```python
from build123d import *

# Parameters (mm, degrees)
SKETCH1_W           = 50.8
SKETCH1_H           = 39.878
BOSS_EXTRUDE1_DEPTH = 53.499926347
SKETCH3_W           = 43.18
SKETCH3_H           = 50.8
CUT_EXTRUDE1_DEPTH  = 30.353
CUT_EXTRUDE2_DEPTH  = 51.8
FILLET3_R           = 2.54
FILLET4_R           = 2.54
FILLET5_R           = 2.54
SKETCH5_R           = 3.175
CUT_EXTRUDE3_DEPTH  = 6.08
CUT_EXTRUDE4_DEPTH  = 25.4


with BuildPart() as part:
    # Sketch1 → Boss-Extrude1 (new body)
    with BuildSketch(Plane(origin=(0, 0, 0), x_dir=(1, 0, 0), z_dir=(0, 1, 0))):
        with Locations((25.4, 19.939)):
            Rectangle(SKETCH1_W, SKETCH1_H)
    extrude(amount=BOSS_EXTRUDE1_DEPTH)

    # Sketch3 → Cut-Extrude1 (cut)
    with BuildSketch(Plane.XY):
        with Locations((25.4, 30.48)):
            Rectangle(SKETCH3_W, SKETCH3_H)
    extrude(amount=-CUT_EXTRUDE1_DEPTH, mode=Mode.SUBTRACT)

    # Sketch4 → Cut-Extrude2 (cut, through all)
    with BuildSketch(Plane.ZY):
        Polygon((0, 18.701926347), (-28.067, 53.499926347), (0, 53.499926347), align=None)
    extrude(amount=-CUT_EXTRUDE2_DEPTH, mode=Mode.SUBTRACT)

    # Fillet3
    fillet3_edges = [part.edges().sort_by_distance(p)[0] for p in [
        (25.4, 53.499926347, -39.878),
    ]]
    fillet(fillet3_edges, radius=FILLET3_R)

    # Fillet4
    fillet4_edges = [part.edges().sort_by_distance(p)[0] for p in [
        (48.895, 53.499926347, -28.067),
        (1.905, 53.499926347, -28.067),
    ]]
    fillet(fillet4_edges, radius=FILLET4_R)

    # Fillet5
    fillet5_edges = [part.edges().sort_by_distance(p)[0] for p in [
        (50.8, 0, -19.939),
        (0, 0, -19.939),
    ]]
    fillet(fillet5_edges, radius=FILLET5_R)

    # Sketch5 → Cut-Extrude3 (cut, through all)
    with BuildSketch(Plane(origin=(0, 5.08, 0), x_dir=(1, 0, 0), z_dir=(0, 1, 0))):
        with Locations((23.622, 6.35)):
            Circle(SKETCH5_R)
        with Locations((23.622, 24.003)):
            Circle(SKETCH5_R)
    extrude(amount=-CUT_EXTRUDE3_DEPTH, mode=Mode.SUBTRACT)

    # Sketch13 → Cut-Extrude4 (cut)
    with BuildSketch(Plane.XY.offset(-30.353)):
        with BuildLine():
            Line((45.078473315, 33.54111133), (45.078473315, 13.162010507))
            Line((45.078473315, 13.162010507), (24.90196768, 10.132947276))
            ThreePointArc((24.90196768, 10.132947276), (7.104992388, 24.03759453), (24.712163172, 38.181818856))
            Line((24.712163172, 38.181818856), (45.078473315, 33.54111133))
        make_face()
    extrude(amount=-CUT_EXTRUDE4_DEPTH, mode=Mode.SUBTRACT)


solid = part.part
```
Check sheet for the modelled part. Datum: model origin and axes. Units: mm. A direction names the side the tool comes from. Give positions to 0.01 mm unless a question says otherwise; leave off trailing zeros. Write each loop counter-clockwise with the first axis right and the second up, starting at its lowest first coordinate (ties: lowest second). Pieces come first, ordered by that corner, then holes. Notation, with made-up numbers: (-24, 49.5) -> (15, 49.5) arc R13 cw to (15, 73.5) -> close; hole circle Ø6 at (3, 38). An arc over 180 degrees is marked (long way). Use CSV: the item, a comma, the result in double quotes. Start each with the question number.
Q1. Tool access check on faces 1 (the flat face through (34.753, 35.894, -35.049)), 2 (the flat face through (50.8, 22, -24)), 3 (the flat face through (25, 40, -30.353)). Record the directions out of +Z, -Z, +X, -X, +Y, -Y that give a thin tool (end or side, any length) a straight path to the whole face; none if there is none.
Q2. Cross-section at C-C on z = -4. Enter the section's corners in (x, y), and give its area (3 significant figures).
Q3. Cross-section at D-D on z = -19. Enter the section's corners in (x, y).
Q4. Cross-section at A-A on y = 26. Enter the section's corners in (x, z), and give its area (3 significant figures).
Q5. Release check for a two-part mould opening along Y. For faces 4 (the flat face through (25, 0, -20)), 5 (the flat face through (25, 53.5, -33)), 6 (the flat face through (35.13, 11.67, -35.05)), 7 (the cylindrical face through (26.65, 2.58, -7.3)) record: +Y half, -Y half, draft (parallel to the pull), parting line (faces both ways), or undercut.
Q6. Depth check by flat-ended pin: P1, Ø9, axis at x = 34, z = -16, coming from the +Y side; P2, Ø1.5, axis at x = 21.5, z = -16, coming from the -Y side; P3, Ø1.5, axis at x = 40.5, y = 8.5, coming from the +Z side. Enter the tip coordinate at first touch or a pass-through.
Q7. Cross-section at B-B on x = 17. Enter the section's corners in (y, z), and give its area (3 significant figures).
Q8. Scan lines: line 1 along X through (y, z) = (9.5, -11); line 2 along Y through (x, z) = (15, -35); line 3 along Y through (x, z) = (27, -9). Record each from-to range of solid material in increasing order.
Working result:
1,face 1,"+Z, -Z"
1,face 2,"+Z, -Z, +X, +Y, -Y"
1,face 3,"+Z, +Y"
2,outline,"(0, 2.54) arc R2.54 ccw to (2.54, 0) -> (21.49, 0) -> (21.49, 5.08) -> (3.81, 5.08) -> (3.81, 23.66) -> (0, 23.66) -> close; (25.76, 0) -> (48.26, 0) arc R2.54 ccw to (50.8, 2.54) -> (50.8, 23.66) -> (46.99, 23.66) -> (46.99, 5.08) -> (25.76, 5.08) -> close"
2,area,"375 mm^2"
3,outline,"(0, 2.54) arc R2.54 ccw to (2.54, 0) -> (48.26, 0) arc R2.54 ccw to (50.8, 2.54) -> (50.8, 42.26) -> (46.99, 42.26) -> (46.99, 5.08) -> (3.81, 5.08) -> (3.81, 42.26) -> (0, 42.26) -> close"
4,outline,"(0, -39.88) -> (7.23, -39.88) -> (7.23, -30.35) -> (3.81, -30.35) -> (3.81, -5.89) -> (0, -5.89) -> close; (45.08, -39.88) -> (50.8, -39.88) -> (50.8, -5.89) -> (46.99, -5.89) -> (46.99, -30.35) -> (45.08, -30.35) -> close"
4,area,"310 mm^2"
5,face 4,"-Y half"
5,face 5,"+Y half"
5,face 6,"undercut"
5,face 7,"draft"
6,P1,"stops at y = 5.08"
6,P2,"stops at y = 0"
6,P3,"stops at z = -30.35"
7,outline,"(0, -39.88) -> (10.45, -39.88) -> (10.45, -30.35) -> (5.08, -30.35) -> (5.08, 0) -> (0, 0) -> close; (37.82, -39.88) -> (50.96, -39.88) arc R2.54 ccw to (53.5, -37.34) -> (53.5, -30.35) -> (37.82, -30.35) -> close"
7,area,"402 mm^2"
8,line 1,"x = 0 to 3.81, 46.99 to 50.8"
8,line 2,"y = 0 to 11.28, 36.99 to 53.5"
8,line 3,"y = 0 to 5.08"
